Could you check a few things on this model? Use its own coordinates, in mm. A direction names the side the tool comes from. Round coordinates to 2 decimals unless told otherwise and drop trailing zeros. Order: outer loops, then holes, each group sorted by start corner. A loop starts at its lowest first (then second) coordinate and runs counter-clockwise, first axis right, second up. Notation, with made-up numbers: M 74.5,74 L 85.5,74 A23 ccw 85.5,108 Z; hole C 71,34 d5. An arc over 180 degrees is marked long. Write each question's results on one line, items separated by ' | '. Start each with the question number.
1. For faces 3 (the cylindrical face through (-5.506, -27.287, -24.796)), 4 (the flat face through (24.5, -26.035, -8.1)), which set-ups out of +Z, -Z, +X, -X, +Y, -Y let a thin tool reach every point of the face, with its end or its side?
2. Suppose I cut it at B-B on z = 0. Write out the boundary of the cut face in (x, y) (3 decimals).
3. Please list where these lines run through material, in increasing order: L1, parallel to Z at x = -8, y = -17; L2, parallel to X at y = -3, z = -17.5; L3, parallel to Z at x = 0, y = -21.
4. Suppose I cut it at C-C on y = -7.25. Write out the boundary of the cut face in (x, z), and give its area (3 significant figures).
5. We'd pull the mould along Y, two halves only. Please class faces 1 (the cylindrical face through (-3.932, -14.158, 29.947)), 2 (the cylindrical face through (-5.997, -14.123, -27.007)): released by +Y, released by -Y, zero draft, split by the parting line, or undercut.
6. Suppose I cut it at D-D on y = -24.5. Write out the boundary of the cut face in (x, z), and give its area (3 significant figures).
7. Suppose I cut it at A-A on x = 0. Write out the boundary of the cut face in (y, z) (3 decimals), and give its area (3 significant figures).
8. I'm going to push flat-ended pins straight in: pin 1 (1.5 mm diameter, centred on y = -9, z = 14, fed in from -X); pin 2 (5 mm diameter, centred on y = -22, z = -14.5, fed in from +X); pin 3 (10 mm diameter, centred on x = -17, y = -11.5, fed in from +Z). Where does each tip first touch, or does it pass through?
from build123d import *

# Parameters (mm, degrees)
F0_R     = 30.20441
F0_R_2   = 25.4
F2_DEPTH = 28.575
F3_T     = -2.54


# Not quite as in the source:
# - a fillet or chamfer that OpenCascade refuses, or shapes differently, is made with other operations: its cross-section is extruded or revolved along the edge and cut away or added


with BuildPart() as f2:
    # F0 (on Front) → F2 (new body)
    with BuildSketch(Plane.XZ):
        Circle(F0_R)
        Circle(F0_R_2, mode=Mode.SUBTRACT)
    extrude(amount=F2_DEPTH)

    # F3
    f3_openings = [f2.faces().sort_by_distance(p)[0] for p in [
        (-25.4, -14.2875, 0),
    ]]
    offset(amount=F3_T, openings=f3_openings)

    # F4: fillet of radius 5.08 on 2 edges, made by hand

    # F4_s1 → F4_t2 (revolve, cut)
    with BuildSketch(Plane.XY):
        with BuildLine():
            ThreePointArc((30.20441, -5.072519113), (28.8126614285, -1.5792110247), (25.4, 0))
            Line((25.4, 0), (30.20441, 0))
            Line((30.20441, 0), (30.20441, -5.072519113))
        make_face()
    revolve(axis=Axis((0, 0, 0), (0, -1, 0)), mode=Mode.SUBTRACT)

    # F4_s3 → F4_t4 (revolve, cut)
    with BuildSketch(Plane.XY):
        with BuildLine():
            ThreePointArc((30.20441, -23.502480887), (28.8126614285, -26.9957889753), (25.4, -28.575))
            Line((25.4, -28.575), (30.20441, -28.575))
            Line((30.20441, -28.575), (30.20441, -23.502480887))
        make_face()
    revolve(axis=Axis((0, -28.575, 0), (0, -1, 0)), mode=Mode.SUBTRACT)


solid = f2.part
Filled sheet:
1) face 3: +Y, -Y | face 4: none
2) outline: M -30.204,-23.502 A5.08 ccw -25.4,-28.575 L -25.4,-26.035 L -27.664,-26.035 L -27.664,-2.54 L -25.4,-2.54 L -25.4,0 A5.08 ccw -30.204,-5.073 Z; M 25.4,-28.575 A5.08 ccw 30.204,-23.502 L 30.204,-5.073 A5.08 ccw 25.4,0 L 25.4,-2.54 L 27.664,-2.54 L 27.664,-26.035 L 25.4,-26.035 Z
3) L1: z = -29.13 to -26.48, 26.48 to 29.13 | L2: x = -24.07 to -21.43, 21.43 to 24.07 | L3: z = -30.2 to -27.66, 27.66 to 30.2
4) outline: C 0,0 d60.41; hole C 0,0 d55.33 | area: 462 mm^2
5) face 1: zero draft | face 2: undercut
6) outline: C 0,0 d60.21; hole C 0,0 d55.33 | area: 443 mm^2
7) outline: M -28.575,-25.4 A5.08 ccw -23.502,-30.204 L -5.073,-30.204 A5.08 ccw 0,-25.4 L -2.54,-25.4 L -2.54,-27.664 L -26.035,-27.664 L -26.035,-25.4 Z; M -28.575,25.4 L -26.035,25.4 L -26.035,27.664 L -2.54,27.664 L -2.54,25.4 L 0,25.4 A5.08 ccw -5.073,30.204 L -23.502,30.204 A5.08 ccw Z | area: 146 mm^2
8) pin 1: stops at x = -27.14 | pin 2: stops at x = 27.72 | pin 3: stops at z = 27.72
